Model file for the job. Use its own axes, mm. A direction names the side the tool comes from. Round coordinates to 2 decimals unless told otherwise and drop trailing zeros. Write each loop counter-clockwise with the first axis right and the second up, starting at its lowest first coordinate (ties: lowest second). Pieces come first, ordered by that corner, then holes. Notation, with made-up numbers: (71, 69.25) - (86, 69.25) arc R33 cw to (86, 103.25) - close; hole circle Ø11 at (-3, 38.25). An arc over 180 degrees is marked (long way). Answer as a JSON object with one key per item and string values. Group by question number.
from build123d import *

# Parameters (mm, degrees)
SKETCH1_W           = 33.02
SKETCH1_H           = 38.1
BOSS_EXTRUDE1_DEPTH = 2.667
SKETCH2_W           = 14.562666666
SKETCH2_H           = 5.334
SKETCH2_W_2         = 5.334
SKETCH2_H_2         = 12.7
BOSS_EXTRUDE2_DEPTH = 5.334


with BuildPart() as part:
    # Sketch1 → Boss-Extrude1 (new body, symmetric)
    with BuildSketch(Plane(origin=(0, 0, 0), x_dir=(1, 0, 0), z_dir=(0, 1, 0))):
        Rectangle(SKETCH1_W, SKETCH1_H)
    extrude(amount=BOSS_EXTRUDE1_DEPTH, both=True)

    # Sketch2 → Boss-Extrude2 (add)
    with BuildSketch(Plane(origin=(0, 2.667, 0), x_dir=(1, 0, 0), z_dir=(0, 1, 0))):
        with Locations((0, -21.717)):
            Rectangle(SKETCH2_W, SKETCH2_H)
        with Locations((-19.177, 0)):
            Rectangle(SKETCH2_W_2, SKETCH2_H_2)
        with Locations((19.177, 0)):
            Rectangle(SKETCH2_W_2, SKETCH2_H_2)
    extrude(amount=-BOSS_EXTRUDE2_DEPTH)


solid = part.part
(1) Slice it at A-A (y = -0.15). Write the cut outline in (x, z), then the cut area to 3 significant figures.
(2) Slice it at C-C (z = -15). Write the cut outline in (x, y).
(3) Slice it at B-B (x = -8). Write the cut outline in (y, z), then the cut area to 3 significant figures.
(4) Drill centre lines: line 1 (Z direction, x = -14.5, y = 0.65); line 2 (X direction, y = -0.95, z = 8.5); line 3 (Z direction, x = -18.5, y = 1.65). Where is each one in solid material? Low to high. Write a range as from..to.
(5) 3-axis set-ups, long thin cutter, end or side, ignore diameter. For faces 1 (the flat face through (-16.51, 0, 13)), 2 (the flat face through (19, 0, -6.35)), 3 (the flat face through (12, 0, 19.05)), 4 (the flat face through (0, 0, 24.384)), 5 (the flat face through (-16.51, 0, -13)): which of +Z, -Z, +X, -X, +Y, -Y reach the whole face in a straight line?
(6) Flat gauge pins, fed straight in: pin 1 (1.6 mm diameter, centred on x = -11, y = -1, fed in from +Z); pin 2 (1.6 mm diameter, centred on x = -18, y = 0.5, fed in from +Z); pin 3 (2.5 mm diameter, centred on y = 1, z = 12, fed in from +X). Where does each tip first touch, or does it go through?
Answer:
{
 "1": {"outline": "(-21.84, -6.35) - (-16.51, -6.35) - (-16.51, -19.05) - (16.51, -19.05) - (16.51, -6.35) - (21.84, -6.35) - (21.84, 6.35) - (16.51, 6.35) - (16.51, 19.05) - (7.28, 19.05) - (7.28, 24.38) - (-7.28, 24.38) - (-7.28, 19.05) - (-16.51, 19.05) - (-16.51, 6.35) - (-21.84, 6.35) - close", "area": "1,470 mm²"},
 "2": {"outline": "(-16.51, -2.67) - (16.51, -2.67) - (16.51, 2.67) - (-16.51, 2.67) - close"},
 "3": {"outline": "(-2.67, -19.05) - (2.67, -19.05) - (2.67, 19.05) - (-2.67, 19.05) - close", "area": "203 mm²"},
 "4": {"line 1": "-19.05..19.05", "line 2": "-16.51..16.51", "line 3": "-6.35..6.35"},
 "5": {"face 1": "+Z, -X, +Y, -Y", "face 2": "-Z, +X, +Y, -Y", "face 3": "+Z, +X, +Y, -Y", "face 4": "+Z, +X, -X, +Y, -Y", "face 5": "-Z, -X, +Y, -Y"},
 "6": {"pin 1": "z = 19.05", "pin 2": "z = 6.35", "pin 3": "x = 16.51"}
}
